from build123d import *

# Parameters (mm, degrees)
SKETCH1_W               = 50.8
SKETCH1_H               = 50.8
SKETCH1_W_2             = 47.625
SKETCH1_H_2             = 47.625
BOSS_EXTRUDE1_DEPTH     = 254
SKETCH6_R               = 2.3999952
CUT_EXTRUDE3_DEPTH      = 1
CUT_EXTRUDE3_DEPTH_BACK = 51.8
SKETCH7_R               = 2.3999952
CUT_EXTRUDE4_DEPTH      = 1
CUT_EXTRUDE4_DEPTH_BACK = 51.8
SKETCH8_R               = 1.8034
CUT_EXTRUDE5_DEPTH      = 51.8
SKETCH9_R               = 1.8034
CUT_EXTRUDE6_DEPTH      = 51.8
SKETCH10_W              = 44.45
SKETCH10_H              = 1.5875
CUT_EXTRUDE7_DEPTH      = 51.8


with BuildPart() as part:
    # Sketch1 → Boss-Extrude1 (new body)
    with BuildSketch(Plane(origin=(0, 0, 0), x_dir=(1, 0, 0), z_dir=(0, 1, 0))):
        Rectangle(SKETCH1_W, SKETCH1_H)
        Rectangle(SKETCH1_W_2, SKETCH1_H_2, mode=Mode.SUBTRACT)
    extrude(amount=BOSS_EXTRUDE1_DEPTH)

    # Sketch6 → Cut-Extrude3 (cut, two sides)
    with BuildSketch(Plane(origin=(25.4, 0, 0), x_dir=(0, 0, -1), z_dir=(1, 0, 0))) as cut_extrude3_sk:
        with Locations((0, 12.412400118)):
            Circle(SKETCH6_R)
    extrude(amount=CUT_EXTRUDE3_DEPTH, mode=Mode.SUBTRACT)
    extrude(cut_extrude3_sk.sketch, amount=-CUT_EXTRUDE3_DEPTH_BACK, mode=Mode.SUBTRACT)

    # Sketch7 → Cut-Extrude4 (cut, two sides)
    with BuildSketch(Plane(origin=(0, 0, -25.4), x_dir=(-1, 0, 0), z_dir=(0, 0, -1))) as cut_extrude4_sk:
        with Locations((0, 12.412400118)):
            Circle(SKETCH7_R)
    extrude(amount=CUT_EXTRUDE4_DEPTH, mode=Mode.SUBTRACT)
    extrude(cut_extrude4_sk.sketch, amount=-CUT_EXTRUDE4_DEPTH_BACK, mode=Mode.SUBTRACT)

    # Sketch8 → Cut-Extrude5 (cut, through all)
    with BuildSketch(Plane(origin=(25.4, 0, 0), x_dir=(0, 0, -1), z_dir=(1, 0, 0))):
        with Locations((0, 247.65)):
            Circle(SKETCH8_R)
    extrude(amount=-CUT_EXTRUDE5_DEPTH, mode=Mode.SUBTRACT)

    # Sketch9 → Cut-Extrude6 (cut, through all)
    with BuildSketch(Plane.XY.offset(25.4)):
        with Locations((0, 247.65)):
            Circle(SKETCH9_R)
    extrude(amount=-CUT_EXTRUDE6_DEPTH, mode=Mode.SUBTRACT)

    # Sketch10 → Cut-Extrude7 (cut, through all)
    with BuildSketch(Plane.XY.offset(25.4)):
        with Locations((0, 152.4)):
            Rectangle(SKETCH10_W, SKETCH10_H)
    extrude(amount=-CUT_EXTRUDE7_DEPTH, mode=Mode.SUBTRACT)


solid = part.part
Can you work these out from the model? Positions are in its coordinate system, mm. A direction names the side the tool comes from. Give positions to 0.01 mm unless a question says otherwise; leave off trailing zeros. Loops run counter-clockwise (first coordinate to the right, second up) from the corner with the lowest first, then second, coordinate; pieces in that order, holes last. Notation, with made-up numbers: (29, 44.5) -> (44, 44.5) arc R19 ccw to (44, 64.5) -> close; hole circle Ø6 at (68, 41). An arc over 180 degrees is marked (long way). Write item = value, one per line.
1) Suppose I cut it at C-C on y = 233.5. Write out the boundary of the cut face in (x, z).
Check result:
outline = (-25.4, -25.4) -> (25.4, -25.4) -> (25.4, 25.4) -> (-25.4, 25.4) -> close; hole (-23.81, -23.81) -> (23.81, -23.81) -> (23.81, 23.81) -> (-23.81, 23.81) -> close
2) Thinking about a two-plate mould opening in Z: for faces 1 (the flat face through (0, 125, 25.4)), 2 (the flat face through (-2, 0, 24)), 3 (the flat face through (0, 125, -23.812)), 4 (the cylindrical face through (-24.6, 13.1, -2.3)), which applies, released by +Z, released by -Z, zero draft, split by the parting line, or undercut?
Check result:
face_1 = released by +Z
face_2 = zero draft
face_3 = undercut
face_4 = undercut
3) For faces 5 (the cylindrical face through (24.6, 13.1, -2.3)), 6 (the flat face through (-23.812, 125, 0)), which set-ups out of +Z, -Z, +X, -X, +Y, -Y let a thin tool reach every point of the face, with its end or its side?
Check result:
face_5 = +X, -X
face_6 = +Y, -Y
4) Suppose I cut it at A-A on z = 16. Write out the boundary of the cut face in (x, y).
Check result:
outline = (-25.4, 0) -> (-23.81, 0) -> (-23.81, 254) -> (-25.4, 254) -> close; (23.81, 0) -> (25.4, 0) -> (25.4, 254) -> (23.81, 254) -> close
5) I need wall thicknesses on L1, parallel to Y at x = 0, z = 24.1; L2, parallel to Y at x = 24, z = 0; L3, parallel to X at y = 89.5, z = 11. Which ranges of each line are inside material? Lowest first, please. Write a range as from..to.
Check result:
L1 = 0..10.01, 14.81..151.61, 153.19..245.85, 249.45..254
L2 = 0..10.01, 14.81..245.85, 249.45..254
L3 = -25.4..-23.81, 23.81..25.4
6) Suppose I cut it at B-B on x = -17.5. Write out the boundary of the cut face in (y, z).
Check result:
outline = (0, -25.4) -> (151.61, -25.4) -> (151.61, -23.81) -> (0, -23.81) -> close; (0, 23.81) -> (151.61, 23.81) -> (151.61, 25.4) -> (0, 25.4) -> close; (153.19, -25.4) -> (254, -25.4) -> (254, -23.81) -> (153.19, -23.81) -> close; (153.19, 23.81) -> (254, 23.81) -> (254, 25.4) -> (153.19, 25.4) -> close
